Job drawing, mm, ordinate dimensions from the low corner. One solid piece. A direction names the side the tool comes from. Round coordinates to 2 decimals unless told otherwise and drop trailing zeros. Order: outer loops, then holes, each group sorted by start corner. A loop starts at its lowest first (then second) coordinate and runs counter-clockwise, first axis right, second up. Notation, with made-up numbers: (-28.75, 5) -> (-4.75, 5) arc R23 cw to (-4.75, 33) -> close; hole circle Ø9 at (-22, 16.5). An arc over 180 degrees is marked (long way). Return JSON: item names as keys, results as strings. Group by question number.
Q1. Mould opens along Z. For the marked faces 1, 2 and 3 say: +Z half, -Z half, draft (parallel to the pull), parting line (faces both ways), or undercut.
Q2. Flat gauge pins, fed straight in: pin 1 (5 mm diameter, centred on x = 20, y = 112, fed in from -Z); pin 2 (4 mm diameter, centred on x = 11.5, y = 125.5, fed in from -Z). Where does each tip first touch, or does it go through?
Q3. Cut at C-C (z = 110). Write the cut outline in (x, y) (1 decimal), then the cut area to 3 significant figures.
Q4. Probe line 1 along Y through (x, z) = (25, 129) (1 decimal); line 2 along Z through (x, y) = (30.5, 182); line 3 along Z through (x, y) = (28, 20) (1 decimal). List the from-to ranges inside material, lowest first.
Q5. Which spindle directions (+Z, -Z, +X, -X, +Y, -Y) get a long thin tool onto all of the face, cutting with end or side? Do the marked faces 4 and 5. Say none if no direction does.
Q6. Cut at B-B (y = 95). Write the cut outline in (x, z) (1 decimal), then the cut area to 3 significant figures.
Q7. Cut at D-D (z = 138). Write the cut outline in (x, y).
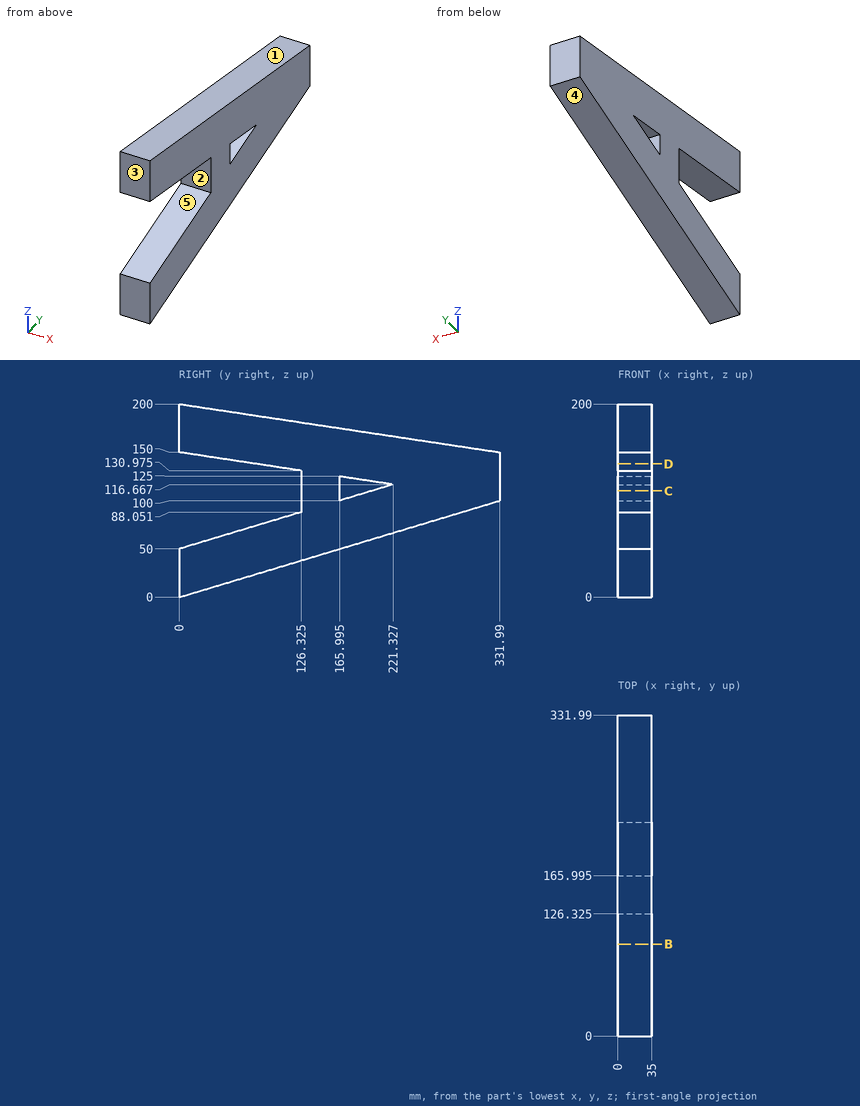
Solution:
{
 "1": {"face 1": "+Z half", "face 2": "undercut", "face 3": "draft"},
 "2": {"pin 1": "stops at z = 32.98", "pin 2": "stops at z = 37.2"},
 "3": {"outline": "(0, 126.3) -> (35, 126.3) -> (35, 166) -> (0, 166) -> close; (0, 199.2) -> (35, 199.2) -> (35, 332) -> (0, 332) -> close", "area": "6,040 mm²"},
 "4": {"line 1": "y = 126.3 to 332", "line 2": "z = 54.82 to 104.82, 122.59 to 172.59", "line 3": "z = 6 to 56, 147 to 197"},
 "5": {"face 4": "-Z, +X, -X, +Y", "face 5": "+X, -X, -Y"},
 "6": {"outline": "(0, 28.6) -> (35, 28.6) -> (35, 78.6) -> (0, 78.6) -> close; (0, 135.7) -> (35, 135.7) -> (35, 185.7) -> (0, 185.7) -> close", "area": "3,500 mm²"},
 "7": {"outline": "(0, 79.68) -> (35, 79.68) -> (35, 331.99) -> (0, 331.99) -> close"}
}
